from build123d import *

# Parameters (mm, degrees)
BOSS_EXTRUDE3_DEPTH   = 1100
SKETCH2_4_R           = 8
BOSS_EXTRUDE4_DEPTH   = 1100
F_5_0MM_DOWEL_HOLE1_D = 5
LPATTERN1_COUNT       = 8
LPATTERN1_PITCH       = 150


with BuildPart() as part:
    # Sketch2 → Boss-Extrude3 (new body)
    with BuildSketch(Plane.XY):
        with BuildLine():
            Line((-20, 5), (-20, 0))
            Line((-20, 0), (20, 0))
            Line((20, 0), (20, 5))
            Line((20, 5), (8, 5))
            Line((8, 5), (8, 10))
            Line((8, 10), (3.872983346, 18))
            ThreePointArc((3.872983346, 18), (0, 17), (-3.872983346, 18))
            Line((-3.872983346, 18), (-8, 10))
            Line((-8, 10), (-8, 5))
            Line((-8, 5), (-20, 5))
        make_face()
    extrude(amount=BOSS_EXTRUDE3_DEPTH)

    # Sketch2_4 → Boss-Extrude4 (add)
    with BuildSketch(Plane.XY):
        with Locations((0, 25)):
            Circle(SKETCH2_4_R)
    extrude(amount=BOSS_EXTRUDE4_DEPTH)

    # 5.0mm Dowel Hole1 (through all)
    with Locations(Plane(origin=(0, 5, 0), x_dir=(1, 0, 0), z_dir=(0, 1, 0))):
        with Locations((15, -1075), (-15, -1075)):
            f_5_0mm_dowel_hole1 = Hole(F_5_0MM_DOWEL_HOLE1_D / 2)

    # LPattern1: 5.0mm Dowel Hole1 ×8
    with Locations(*[(0, 0, -i * LPATTERN1_PITCH) for i in range(1, LPATTERN1_COUNT)]):
        add(f_5_0mm_dowel_hole1, mode=Mode.SUBTRACT)


solid = part.part
Model file for the job. Use its own axes, mm. Coordinates: 2 decimals unless noted, no trailing zeros. Order: outer loops, then holes, each group sorted by start corner. A loop starts at its lowest first (then second) coordinate and runs counter-clockwise, first axis right, second up. Notation, with made-up numbers: M 55,-24.5 L 89,-24.5 A31 ccw 89,11.5 Z; hole C -19,-9.5 d4. An arc over 180 degrees is marked long. Return JSON: item names as keys, results as strings.
1. Drill centre lines: probe 1 along X at (y, z) = (2.4, 1075); probe 2 along Y at (x, z) = (-10.5, 616); probe 3 along X at (y, z) = (25, 344). Where is each one in solid material? Low to high.
Ans:
{"probe 1": "-20 to -17.5, -12.5 to 12.5, 17.5 to 20", "probe 2": "0 to 5", "probe 3": "-8 to 8"}
2. Saw through at A-A (z = 862). Give the cut face in (x, y).
Ans:
{"outline": "M -20,0 L 20,0 L 20,5 L 8,5 L 8,10 L 3.87,18 A8 ccw long -3.87,18 L -8,10 L -8,5 L -20,5 Z"}
3. Flat gauge pins, fed straight in: pin 1 (6.5 mm diameter, centred on x = -15, z = 625, fed in from +Y); pin 2 (1.5 mm diameter, centred on x = 4.5, z = 203.5, fed in from +Y); pin 3 (8 mm diameter, centred on y = 18, z = 370, fed in from +X). Where does each tip first touch, or does it go through?
Ans:
{"pin 1": "y = 5", "pin 2": "y = 32.07", "pin 3": "x = 7.42"}
